Source: CAD feature listing. Evaluate the final solid. Frame: model axes, mm. A direction names the side the tool comes from. Give positions to 0.01 mm unless a question says otherwise; leave off trailing zeros. Write each loop counter-clockwise with the first axis right and the second up, starting at its lowest first coordinate (ties: lowest second). Pieces come first, ordered by that corner, then holes. Notation, with made-up numbers: (61, 55) -> (113, 55) arc R26 cw to (113, 79) -> close; hole circle Ø7 at (1.5, 75). An arc over 180 degrees is marked (long way). Write item = value, one per line.
from build123d import *

# Parameters (mm, degrees)
F0_W     = 35
F0_H     = 25
F2_DEPTH = 3.5
F0_W_2   = 3
F3_DEPTH = 25
F4_DEPTH = 25
F5_D     = 3.4
F5_DEPTH = 20.501
F6_D     = 3.4
F6_DEPTH = 20.501
F7_D     = 3.4


with BuildPart() as f2:
    # F0 (on Top) → F2 (new body)
    with BuildSketch(Plane.XY):
        Rectangle(F0_W, F0_H)
        with BuildLine():
            ThreePointArc((-12.275, 0), (-10.575, 1.7), (-8.875, 0))
            ThreePointArc((-8.875, 0), (-10.575, -1.7), (-12.275, 0))
        make_face(mode=Mode.SUBTRACT)
        with BuildLine():
            ThreePointArc((1.7, 0), (0, -1.7), (-1.7, 0))
            ThreePointArc((-1.7, 0), (0, 1.7), (1.7, 0))
        make_face(mode=Mode.SUBTRACT)
        with BuildLine():
            ThreePointArc((12.275, 0), (10.575, -1.7), (8.875, 0))
            ThreePointArc((8.875, 0), (10.575, 1.7), (12.275, 0))
        make_face(mode=Mode.SUBTRACT)
    extrude(amount=F2_DEPTH)

    # F0 (on Top) → F3 (join)
    with BuildSketch(Plane.XY):
        with Locations((-19, 0)):
            Rectangle(F0_W_2, F0_H)
    extrude(amount=F3_DEPTH)

    # F0 (on Top) → F4 (join)
    with BuildSketch(Plane.XY):
        with Locations((19, 0)):
            Rectangle(F0_W_2, F0_H)
    extrude(amount=F4_DEPTH)

    # F5 (through all, one way)
    with BuildSketch(Plane(origin=(0, 0, 0), x_dir=(0, 1, 0), z_dir=(-1, 0, 0))):
        with Locations((-9.9837460197, -21.689)):
            Circle(F5_D / 2)
    extrude(amount=-F5_DEPTH, mode=Mode.SUBTRACT)

    # F6 (through all, one way)
    with BuildSketch(Plane(origin=(0, 0, 0), x_dir=(0, 1, 0), z_dir=(-1, 0, 0))):
        with Locations((10.6162539803, -21.689)):
            Circle(F6_D / 2)
    extrude(amount=-F6_DEPTH, mode=Mode.SUBTRACT)

    # F7 (through all)
    with Locations(Plane.YZ):
        with Locations((-9.9837460197, 21.689), (10.6162539803, 21.689)):
            Hole(F7_D / 2)


solid = f2.part
1) Access query for faces 1 (the flat face through (0, 3, 3.5)), 2 (the cylindrical face through (0.37, -1.66, 1.73)). Directions: +Z, -Z, +X, -X, +Y, -Y. A direction counts if a zero-diameter tool reaches every point of the face in a straight line with its end or side. Return the directions, or none.
Computed:
face_1 = +Z, +Y, -Y
face_2 = +Z, -Z
2) Cut plane B-B (x = 0). Return the cut outline in (y, z), then the cut area to 3 significant figures.
Computed:
outline = (-12.5, 0) -> (-1.7, 0) -> (-1.7, 3.5) -> (-12.5, 3.5) -> close; (1.7, 0) -> (12.5, 0) -> (12.5, 3.5) -> (1.7, 3.5) -> close
area = 75.6 mm²
3) Contact query for flat-ended pins moving along their axis: pin 1 (1 mm diameter, centred on x = 12.5, y = -9, fed in from +Z); pin 2 (3 mm diameter, centred on x = 0, y = 0, fed in from +Z). Output: stop coordinate, or through.
Computed:
pin_1 = 3.5
pin_2 = through
4) Cut plane A-A (z = 8). Return the cut outline in (x, y), then the cut area to 3 significant figures.
Computed:
outline = (-20.5, -12.5) -> (-17.5, -12.5) -> (-17.5, 12.5) -> (-20.5, 12.5) -> close; (17.5, -12.5) -> (20.5, -12.5) -> (20.5, 12.5) -> (17.5, 12.5) -> close
area = 150 mm²
5) Cut plane C-C (y = 0). Return the cut outline in (x, z) (3 decimals).
Computed:
outline = (-20.5, 0) -> (-12.275, 0) -> (-12.275, 3.5) -> (-17.5, 3.5) -> (-17.5, 25) -> (-20.5, 25) -> close; (-8.875, 0) -> (-1.7, 0) -> (-1.7, 3.5) -> (-8.875, 3.5) -> close; (1.7, 0) -> (8.875, 0) -> (8.875, 3.5) -> (1.7, 3.5) -> close; (12.275, 0) -> (20.5, 0) -> (20.5, 25) -> (17.5, 25) -> (17.5, 3.5) -> (12.275, 3.5) -> close
6) Draft query along X for faces 3 (the flat face through (20.5, 0, 12)), 4 (the flat face through (0, 3, 0)), 5 (the flat face through (-17.5, 0, 14)). Return one class per face: pulls with the +X half, pulls with the -X half, needs draft (parallel to the pull), parting line crosses it, or undercut.
Computed:
face_3 = pulls with the +X half
face_4 = needs draft
face_5 = undercut
7) Cut plane D-D (y = -3.5). Return the cut outline in (x, z), then the cut area to 4 significant figures.
Computed:
outline = (-20.5, 0) -> (20.5, 0) -> (20.5, 25) -> (17.5, 25) -> (17.5, 3.5) -> (-17.5, 3.5) -> (-17.5, 25) -> (-20.5, 25) -> close
area = 272.5 mm²
8) Material intervals for L1, parallel to X at y = -2.5, z = 15; L2, parallel to Z at x = -8, y = -7.5, sorted ascending.
Computed:
L1 = -20.5 to -17.5, 17.5 to 20.5
L2 = 0 to 3.5
